Design review of the part shown in the three views and the two pictorial views. Dimensions are in mm from the part's minimum x, y and z. A direction names the side the tool comes from. Round coordinates to 2 decimals unless told otherwise and drop trailing zeros. Loops run counter-clockwise (first coordinate to the right, second up) from the corner with the lowest first, then second, coordinate; pieces in that order, holes last. Notation, with made-up numbers: (-10, 53.25) -> (20, 53.25) arc R16 ccw to (20, 75.25) -> close; hole circle Ø9 at (-0.5, 49.25). An arc over 180 degrees is marked (long way). Use CSV: the item, a comma, the result in double quotes. Start each with the question number.
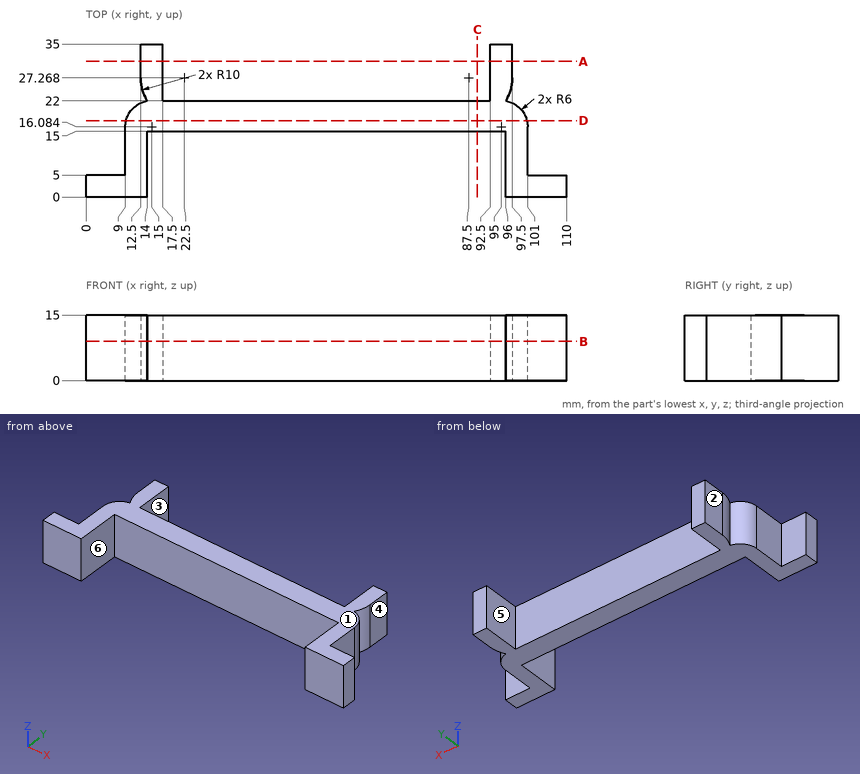
1. For line 1 along X through (y, z) = (27.5, 12); line 2 along X through (y, z) = (13.5, 7.25); line 3 along Y through (x, z) = (49, 2.5), list the stretches that pass through material, from the lowest coordinate up. Write a range as from..to.
2. Clearance check with flat-ended pins moving along their axes: P1, Ø2, axis at x = 29.5, z = 10.5, coming from the +Y side; P2, Ø6, axis at y = 32.5, z = 9, coming from the -X side; P3, Ø8.5, axis at y = 29.5, z = 5, coming from the +X side. State where each tip first meets the part, or that it passes through.
3. Take a section at C-C, the plane x = 89.5. Give the boundary of the cut face in (y, z), then the cut area to 3 significant figures.
4. Take a section at A-A, the plane y = 31. Give the boundary of the cut face in (x, z), then the cut area to 3 significant figures.
5. Take a section at D-D, the plane y = 17.5. Give the boundary of the cut face in (x, z).
6. Take a section at B-B, the plane z = 9. Give the boundary of the cut face in (x, y), then the cut area to 3 significant figures.
7. For the marked faces 4, 5 and 6, list the 3-axis set-ups (+Z, -Z, +X, -X, +Y, -Y) from which the entire face can be reached by the end or side of a thin tool; tool diameter is ignored.
8. The part is to be moulded in two halves that separate along X. For the marked faces 1, 2 and 3, say which applies: pulls with the +X half, pulls with the -X half, needs draft (parallel to the pull), parting line crosses it, or undercut.
Results:
1,line 1,"12.5..17.5, 92.5..97.5"
1,line 2,"9..14, 96..101"
1,line 3,"15..22"
2,P1,"y = 22"
2,P2,"x = 12.5"
2,P3,"x = 97.5"
3,outline,"(15, 0) -> (22, 0) -> (22, 15) -> (15, 15) -> close"
3,area,"105 mm²"
4,outline,"(12.5, 0) -> (17.5, 0) -> (17.5, 15) -> (12.5, 15) -> close; (92.5, 0) -> (97.5, 0) -> (97.5, 15) -> (92.5, 15) -> close"
4,area,"150 mm²"
5,outline,"(9.17, 0) -> (100.83, 0) -> (100.83, 15) -> (9.17, 15) -> close"
6,outline,"(0, 0) -> (14, 0) -> (14, 15) -> (96, 15) -> (96, 0) -> (110, 0) -> (110, 5) -> (101, 5) -> (101, 16.08) arc R6 ccw to (96, 22) arc R10 ccw to (97.5, 27.27) -> (97.5, 35) -> (92.5, 35) -> (92.5, 22) -> (17.5, 22) -> (17.5, 35) -> (12.5, 35) -> (12.5, 27.27) arc R10 ccw to (14, 22) arc R6 ccw to (9, 16.08) -> (9, 5) -> (0, 5) -> close"
6,area,"994 mm²"
7,face 4,"+Z, -Z, +X, +Y"
7,face 5,"+Z, -Z, +Y"
7,face 6,"+Z, -Z, -Y"
8,face 1,"needs draft"
8,face 2,"pulls with the -X half"
8,face 3,"undercut"
